The listing builds one solid part. Answer for the finished solid, in the listing's coordinates (mm). A direction names the side the tool comes from. Coordinates: 2 decimals unless noted, no trailing zeros. Order: outer loops, then holes, each group sorted by start corner. A loop starts at its lowest first (then second) coordinate and runs counter-clockwise, first axis right, second up. Notation, with made-up numbers: (61.5, -28.5) -> (74.5, -28.5) arc R16 cw to (74.5, -9.5) -> close; hole circle Ø1 at (5.25, 40.25). An arc over 180 degrees is marked (long way). Return JSON: item names as keys, results as strings.
from build123d import *

# Parameters (mm, degrees)
F0_R      = 60
F1_DEPTH  = 160
F2_R      = 115
F3_DEPTH  = 50
F4_R      = 160
F5_DEPTH  = 18
F6_SIZE   = 5
F7_R      = 42.875
F8_DEPTH  = 86
F9_R      = 27
F10_DEPTH = 430
F11_R     = 91.436725
F12_DEPTH = 25
F13_W     = 16.456575
F13_H     = 102.537059
F14_DEPTH = 25


with BuildPart() as f1:
    # F0 (on Front) → F1 (new body)
    with BuildSketch(Plane.XZ):
        Circle(F0_R)
    extrude(amount=F1_DEPTH)

    # F2 (on face) → F3 (join)
    with BuildSketch(Plane.XZ.offset(160)):
        Circle(F2_R)
    extrude(amount=F3_DEPTH)

    # F4 (on face) → F5 (join)
    with BuildSketch(Plane.XZ.offset(210)):
        Circle(F4_R)
    extrude(amount=F5_DEPTH)

    # F6
    f6_edges = [f1.edges().sort_by_distance(p)[0] for p in [
        (-115, -160, 0),
    ]]
    chamfer(f6_edges, length=F6_SIZE)

    # F7 (on face) → F8 (join)
    with BuildSketch(Plane(origin=(0, 0, 0), x_dir=(-1, 0, 0), z_dir=(0, 1, 0))):
        Circle(F7_R)
    extrude(amount=F8_DEPTH)

    # F9 (on face) → F10 (cut)
    with BuildSketch(Plane(origin=(0, 86, 0), x_dir=(-1, 0, 0), z_dir=(0, 1, 0))):
        Circle(F9_R)
    extrude(amount=-F10_DEPTH, mode=Mode.SUBTRACT)

    # F11 (on face) → F12 (cut)
    with BuildSketch(Plane.XZ.offset(228)):
        Circle(F11_R)
    extrude(amount=-F12_DEPTH, mode=Mode.SUBTRACT)

    # F13 (on Right) → F14 (cut)
    with BuildSketch(Plane.YZ):
        with Locations((-230.708375, 115.195948)):
            Rectangle(F13_W, F13_H)
    extrude(amount=F14_DEPTH, mode=Mode.SUBTRACT)


solid = f1.part
1. Determine the mould class of faces 4 (the face through (-24.93, -187.185, -112.265)), 5 (the face through (12, -222.48, 123)), 6 (the face through (5.85, -56.48, -26.36)) for opening direction Z: pulls with the +Z half, pulls with the -Z half, needs draft (parallel to the pull), parting line crosses it, or undercut.
Answer block:
{"face 4": "parting line crosses it", "face 5": "needs draft", "face 6": "undercut"}
2. The part is cut by section C-C on y = -172.5. Give the vertices of the cut face in (x, z).
Answer block:
{"outline": "circle Ø230 at (0, 0); hole circle Ø54 at (0, 0)"}
3. For faces 1 (the face through (-11.9, -215.68, 90.66)), 2 (the face through (-59.94, -78.88, 2.64)), 3 (the face through (69, -228, -69)), determine the directions among +Z, -Z, +X, -X, +Y, -Y from which every point of the face is accessible in a straight line to the end or side of a thin tool.
Answer block:
{"face 1": "-Y", "face 2": "+Y", "face 3": "+Z, -Z, +X, -X, -Y"}
4. The part is cut by section A-A on z = 0. Give the vertices of the cut face in (x, y) (3 decimals), and give its area (3 significant figures).
Answer block:
{"outline": "(-160, -228) -> (-91.437, -228) -> (-91.437, -203) -> (-27, -203) -> (-27, 86) -> (-42.875, 86) -> (-42.875, 0) -> (-60, 0) -> (-60, -160) -> (-110, -160) -> (-115, -165) -> (-115, -210) -> (-160, -210) -> close; (27, -203) -> (91.437, -203) -> (91.437, -228) -> (160, -228) -> (160, -210) -> (115, -210) -> (115, -165) -> (110, -160) -> (60, -160) -> (60, 0) -> (42.875, 0) -> (42.875, 86) -> (27, 86) -> close", "area": "23,600 mm2"}
5. Consider line 1 (X direction, y = -220.5, z = 0); line 2 (Y direction, x = -99, z = 116.5). Determine where each line is inside the solid, lowest interval first. Write a range as from..to.
Answer block:
{"line 1": "x = -160..-91.44, 91.44..160", "line 2": "y = -228..-210"}
6. The part is cut by section B-B on y = -35. Give the vertices of the cut face in (x, z), and give its area (3 significant figures).
Answer block:
{"outline": "circle Ø120 at (0, 0); hole circle Ø54 at (0, 0)", "area": "9,020 mm2"}
7. Each of these flat-tipped pins is pushed along its axis until it touches: pin 1 Ø6 at (y, z) = (-225, 136.5) entering from +X; pin 2 Ø6 at (x, y) = (5, -141.5) entering from -Z; pin 3 Ø8 at (y, z) = (-128.5, -31) entering from -X. Where does it stop, or does it pass through?
Answer block:
{"pin 1": "stops at x = 88.19", "pin 2": "stops at z = -59.97", "pin 3": "stops at x = -53.58"}
